Could you check a few things on this model? Use its own coordinates, in mm. Face numbers are marked on the shaded views. A direction names the side the tool comes from. Coordinates: 2 decimals unless noted, no trailing zeros. Write each loop counter-clockwise with the first axis right and the second up, starting at its lowest first coordinate (ties: lowest second). Pieces come first, ordered by that corner, then holes.
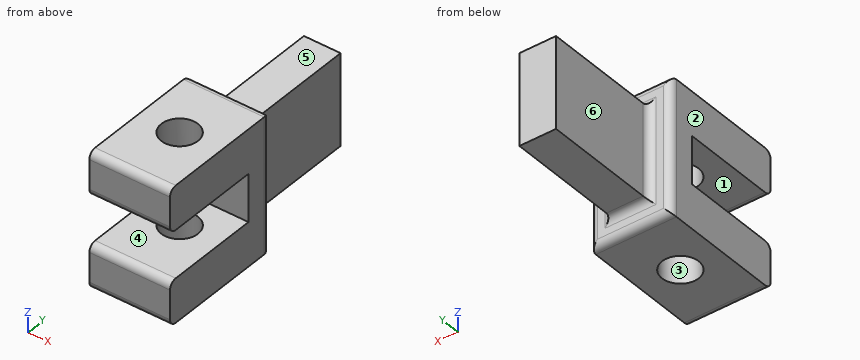
Autodesk Inventor part; units mm, degrees
ref_plane "YZ Plane" through (0, 0, 0) normal (1, 0, 0) x (0, 1, 0)
ref_plane "XZ Plane" through (0, 0, 0) normal (0, 1, 0) x (-1, 0, 0)
ref_plane "XY Plane" through (0, 0, 0) normal (0, 0, 1) x (1, 0, 0)
sketch "Sketch1" plane through (0, 0, 0) normal (1, 0, 0) x (0, 1, 0)
  line L0 (16.25, 12.5) -> (-16.25, 12.5)
  line L1 (-16.25, 12.5) -> (-16.25, -12.5)
  line L2 (-16.25, -12.5) -> (16.25, -12.5)
  line L3 (16.25, -12.5) -> (16.25, 12.5)
  point P0 (0, 0)
  dimension "d0" = 25
  dimension "d1" = 32.5
  dimension "d2" = 16.25
  dimension "d3" = 12.5
extrude "sandwich_plate" add sketch "Sketch1" along normal blind 10
sketch "Sketch2" plane through (0, -16.25, -12.5) normal (0, -1, 0) x (1, 0, 0)
  line L0 (16, -6) -> (-6, -6)
  line L1 (-6, -6) -> (-6, 31)
  line L2 (-6, 31) -> (16, 31)
  line L3 (16, 31) -> (16, -6)
  line L4 (0, 25) -> (10, 25)
  line L5 (0, 0) -> (10, 0)
  line L6 (10, 25) -> (10, 0)
  line L7 (0, 25) -> (0, 0)
  point P0 (0, 12.5)
  dimension "d9" = 6
  dimension "d10" = 6
  dimension "d11" = 6
  dimension "d12" = 6
extrude "clamp_length" add sketch "Sketch2" along normal blind 35 contours L0 L1 L2 L3 | L4 L6 L5 L7
sketch "Sketch3" plane through (16, -16.25, 18.5) normal (1, 0, 0) x (0, 0, -1)
  line L0 (0, -35) -> (37, -35)
  line L1 (12, -35) -> (25, -35)
  line L2 (25, -35) -> (25, -7.5)
  line L3 (25, -7.5) -> (12, -7.5)
  line L4 (12, -7.5) -> (12, -35)
  line L5 (37, 0) -> (0, 0)
  line L6 (0, 0) -> (0, -35)
  line L7 (37, 0) -> (37, -35)
  point P0 (18.5, 16.25)
  dimension "d14" = 7.5
  dimension "d15" = 12
  dimension "d16" = 12
extrude "slot" cut sketch "Sketch3" against normal through all contours L4 L3 L2 L0
fillet "Fillet1" radius 2 12 edges at (5, -16.25, 12.5) (10, -16.25, 0) (0, -16.25, 0) (5, -16.25, -12.5) (16, -16.25, 0) (5, -16.25, 18.5) (-6, -16.25, 0) (5, -16.25, -18.5) (5, -51.25, 6.5) (5, -51.25, -6.5) (5, -51.25, 18.5) (5, -51.25, -18.5)
sketch "Sketch4" plane through (-6, -51.25, 18.5) normal (0, 0, 1) x (1, 0, 0)
  line L0 (22, 33) -> (22, 0)
  line L1 (22, 0) -> (0, 0)
  point P0 (6, 51.25)
  point P1 (11, 17.5)
  dimension "d20" = 11
  dimension "d21" = 17.5
hole "Hole1" at (5, -33.75, 18.5) direction (0, 0, -1) diameter 10 end through all
equation "\"d10\" = d9"
equation "\"d11\" = d9"
equation "\"d12\" = d11"
equation "\"d16\" = d15"
properties part number "support_sandwichPlate" material "Steel, Carbon"
Item 1: If we mould it in two halves opening along X, with no side actions, what happens to the marked faces 1, 2 and 3? For each: released by +X, released by -X, zero draft, split by the parting line, or undercut.
Item 2: I want a section at C-C, the plane x = 5. List the corners of the cut face in (y, z) for me, then the cut area to 3 significant figures.
Item 3: I want a section at B-B, the plane y = -40.5. List the corners of the cut face in (x, z) for me, then the cut area to 3 significant figures.
Item 4: Which directions (+Z, -Z, +X, -X, +Y, -Y) give clear straight access to the entire face, cutting with the end or side of a thin tool? Please do the marked faces 4, 5 and 6.
Item 5: I want a section at D-D, the plane z = 1. List the corners of the cut face in (x, y) for me.
Item 6: Will these pins go through, and if not, where does the flat tip stop? pin 1 Ø20 at (y, z) = (-0.5, -2) entering from +X; pin 2 Ø12 at (x, y) = (0.5, -9) entering from -Z; pin 3 Ø1 at (x, z) = (2.5, -4.5) entering from -Y.
Item 7: I want a section at A-A, the plane y = -33.75. List the corners of the cut face in (x, z) for me.
Item 8: If I drill on line 1 along Z through (x, y) = (13.25, -31); line 2 along Y through (x, z) = (5, -9.75); line 3 along X through (y, z) = (-33.75, -8.75), over which ranges is the centre line in solid material (lowest first)?
Taken from the geometry:
1. face 1: zero draft
1. face 2: released by -X
1. face 3: undercut
2. outline: (-51.25, -16.5) arc R2 ccw to (-49.25, -18.5) - (-38.75, -18.5) - (-38.75, -6.5) - (-49.25, -6.5) arc R2 ccw to (-51.25, -8.5) - close; (-51.25, 8.5) arc R2 ccw to (-49.25, 6.5) - (-38.75, 6.5) - (-38.75, 18.5) - (-49.25, 18.5) arc R2 ccw to (-51.25, 16.5) - close; (-28.75, -18.5) - (-18.25, -18.5) arc R2 ccw to (-16.25, -16.5) - (-16.25, -14.5) arc R2 cw to (-14.25, -12.5) - (16.25, -12.5) - (16.25, 12.5) - (-14.25, 12.5) arc R2 cw to (-16.25, 14.5) - (-16.25, 16.5) arc R2 ccw to (-18.25, 18.5) - (-28.75, 18.5) - (-28.75, 6.5) - (-23.75, 6.5) - (-23.75, -6.5) - (-28.75, -6.5) - close
2. area: 1,510 mm2
3. outline: (-6, -18.5) - (16, -18.5) - (16, -6.5) - (-6, -6.5) - close; (-6, 6.5) - (16, 6.5) - (16, 18.5) - (-6, 18.5) - close
3. area: 528 mm2
4. face 4: +X, -X, -Y
4. face 5: +Z, +X, -X, +Y
4. face 6: +Z, -Z, -X, +Y
5. outline: (-6, -23.75) - (16, -23.75) - (16, -18.25) arc R2 ccw to (14, -16.25) - (12, -16.25) arc R2 cw to (10, -14.25) - (10, 16.25) - (0, 16.25) - (0, -14.25) arc R2 cw to (-2, -16.25) - (-4, -16.25) arc R2 ccw to (-6, -18.25) - close
6. pin 1: stops at x = 10
6. pin 2: stops at z = -12.65
6. pin 3: stops at y = -23.75
7. outline: (-6, -18.5) - (0, -18.5) - (0, -6.5) - (-6, -6.5) - close; (-6, 6.5) - (0, 6.5) - (0, 18.5) - (-6, 18.5) - close; (10, -18.5) - (16, -18.5) - (16, -6.5) - (10, -6.5) - close; (10, 6.5) - (16, 6.5) - (16, 18.5) - (10, 18.5) - close
8. line 1: z = -18.5 to -6.5, 6.5 to 18.5
8. line 2: y = -51.25 to -38.75, -28.75 to 16.25
8. line 3: x = -6 to 0, 10 to 16
